from build123d import *

# Parameters (mm, degrees)
F1_DEPTH       = 20
F3_DEPTH       = 16
F5_DEPTH       = 16
F7_DEPTH       = 16
F9_DEPTH       = 18
F10_R          = 2.5
F11_DEPTH      = 17.4049884739
F11_DEPTH_BACK = 16
F13_DEPTH      = 16


with BuildPart() as f1:
    # F0 (on Top) → F1 (new body)
    with BuildSketch(Plane.XY):
        with BuildLine():
            ThreePointArc((23.6854385647, -8), (24.6691706804, -4.0536425523), (25, 0))
            ThreePointArc((25, 0), (24.6691706804, 4.0536425523), (23.6854385647, 8))
            ThreePointArc((23.6854385647, 8), (17.6776695297, 17.6776695297), (8, 23.6854385647))
            ThreePointArc((8, 23.6854385647), (0, 25), (-8, 23.6854385647))
            ThreePointArc((-8, 23.6854385647), (-17.6776695297, 17.6776695297), (-23.6854385647, 8))
            ThreePointArc((-23.6854385647, 8), (-25, 0), (-23.6854385647, -8))
            ThreePointArc((-23.6854385647, -8), (-17.6776695297, -17.6776695297), (-8, -23.6854385647))
            ThreePointArc((-8, -23.6854385647), (0, -25), (8, -23.6854385647))
            ThreePointArc((8, -23.6854385647), (17.6776695297, -17.6776695297), (23.6854385647, -8))
        make_face()
        with BuildLine():
            ThreePointArc((23.6854385647, 8), (24.6691706804, 4.0536425523), (25, 0))
            ThreePointArc((25, 0), (24.6691706804, -4.0536425523), (23.6854385647, -8))
            Line((23.6854385647, -8), (96.1854385647, -8))
            ThreePointArc((96.1854385647, -8), (104.1854385647, 0), (96.1854385647, 8))
            Line((96.1854385647, 8), (23.6854385647, 8))
        make_face()
        with BuildLine():
            ThreePointArc((-8, 23.6854385647), (0, 25), (8, 23.6854385647))
            Line((8, 23.6854385647), (8, 96.1854385647))
            ThreePointArc((8, 96.1854385647), (0, 104.1854385647), (-8, 96.1854385647))
            Line((-8, 96.1854385647), (-8, 23.6854385647))
        make_face()
        with BuildLine():
            Line((8, -96.1854385647), (8, -23.6854385647))
            ThreePointArc((8, -23.6854385647), (0, -25), (-8, -23.6854385647))
            Line((-8, -23.6854385647), (-8, -96.1854385647))
            ThreePointArc((-8, -96.1854385647), (0, -104.1854385647), (8, -96.1854385647))
        make_face()
        with BuildLine():
            ThreePointArc((-23.6854385647, -8), (-25, 0), (-23.6854385647, 8))
            Line((-23.6854385647, 8), (-96.1854385647, 8))
            ThreePointArc((-96.1854385647, 8), (-104.1854385647, 0), (-96.1854385647, -8))
            Line((-96.1854385647, -8), (-23.6854385647, -8))
        make_face()
    extrude(amount=F1_DEPTH)

    # F2 (on face) → F3 (cut, through all)
    with BuildSketch(Plane.YZ.offset(8)):
        Polygon((104.6854385647, 20), (23.6854385647, 20), (104.6854385647, 3), align=None)
    extrude(amount=-F3_DEPTH, mode=Mode.SUBTRACT)

    # F4 (on face) → F5 (cut, through all)
    with BuildSketch(Plane(origin=(0, 8, 0), x_dir=(-1, 0, 0), z_dir=(0, 1, 0))):
        Polygon((104.6854385647, 20), (23.6854385647, 20), (104.6854385647, 3), align=None)
    extrude(amount=-F5_DEPTH, mode=Mode.SUBTRACT)

    # F6 (on face) → F7 (cut, through all)
    with BuildSketch(Plane(origin=(-8, 0, 0), x_dir=(0, -1, 0), z_dir=(-1, 0, 0))):
        Polygon((104.6854385647, 20), (23.6854385647, 20), (104.6854385647, 3), align=None)
    extrude(amount=-F7_DEPTH, mode=Mode.SUBTRACT)

    # F8 (on face) → F9 (cut)
    with BuildSketch(Plane.XY.offset(20)):
        Polygon((10.7409683065, 0), (-0.5727401924, 11.313708499), (-11.8864486914, 0), (-0.5727401924, -11.313708499), align=None)
    extrude(amount=-F9_DEPTH, mode=Mode.SUBTRACT)

    # F10 (on face) → F11 (cut, two sides)
    with BuildSketch(Plane(origin=(5.3704841533, -5.3704841533, 0), x_dir=(-0.7071067812, -0.7071067812, 0), z_dir=(-0.7071067812, 0.7071067812, 0))) as f11_sk:
        with Locations((0, 3.5)):
            Circle(F10_R)
    extrude(amount=-F11_DEPTH, mode=Mode.SUBTRACT)
    extrude(f11_sk.sketch, amount=F11_DEPTH_BACK, mode=Mode.SUBTRACT)

    # F12 (on face) → F13 (cut, through all)
    with BuildSketch(Plane.XZ.offset(8)):
        Polygon((104.6854385647, 20), (23.6854385647, 20), (104.6854385647, 3), align=None)
    extrude(amount=-F13_DEPTH, mode=Mode.SUBTRACT)


solid = f1.part
CAD build for the part. Positions are in the model's coordinates, mm. A direction names the side the tool comes from. Give positions to 0.01 mm unless a question says otherwise; leave off trailing zeros. Loops run counter-clockwise (first coordinate to the right, second up) from the corner with the lowest first, then second, coordinate; pieces in that order, holes last. Notation, with made-up numbers: M 27.5,9.5 L 55.5,9.5 A14 cw 55.5,14.5 Z; hole C 51.5,-26.75 d5. An arc over 180 degrees is marked long. One line per question, with ' | ' between items. Start each with the question number.
1. 3-axis set-ups, long thin cutter, end or side, ignore diameter. For faces 1 (the face through (8, 51, 8)), 2 (the face through (51, -8, 8)), 3 (the face through (-51, 8, 8)), 4 (the face through (-6.15, 5.736, 10.633)): which of +Z, -Z, +X, -X, +Y, -Y reach the whole face in a straight line?
2. Flat gauge pins, fed straight in: pin 1 (6 mm diameter, centred on x = -50, z = 7, fed in from -Y); pin 2 (6 mm diameter, centred on x = -13, y = -52, fed in from +Z); pin 3 (3 mm diameter, centred on x = 78.5, z = 4, fed in from +Y); pin 4 (10 mm diameter, centred on y = 58.5, z = 6.5, fed in from +X). Where does each tip first touch, or does it go through?
3. Saw through at A-A on z = 17. Give the cut face in (x, y).
4. Saw through at C-C on x = 48. Give the cut face in (y, z).
5. Saw through at B-B on y = 89. Give the cut face in (x, z), plus the area to 3 significant figures.
6. Probe L1, parallel to X at y = -78, z = 8.25; L2, parallel to Y at x = -18, z = 2.5. List the from-to ranges inside material, lowest first. Write a range as from..to.
7. Two-plate mould, pull along Y, no slides. Class faces 5 (the face through (-17.564, 17.791, 9.86)), 6 (the face through (-52, -8, 8)), 7 (the face through (-8, -51, 8)), 8 (the face through (5, -5.74, 11.13)): pulls with the +Y half, pulls with the -Y half, needs draft (parallel to the pull), parting line crosses it, or undercut.
Result sheet:
1) face 1: +Z, -Z, +X, +Y | face 2: +Z, -Z, +X, -Y | face 3: +Z, -Z, -X, +Y | face 4: +Z
2) pin 1: stops at y = -8 | pin 2: passes through | pin 3: stops at y = 8 | pin 4: stops at x = 8
3) outline: M -37.98,-8 L -23.69,-8 A25 ccw -8,-23.69 L -8,-37.98 L 8,-37.98 L 8,-23.69 A25 ccw 23.69,-8 L 37.98,-8 L 37.98,8 L 23.69,8 A25 ccw 8,23.69 L 8,37.98 L -8,37.98 L -8,23.69 A25 ccw -23.69,8 L -37.98,8 Z; hole M -11.89,0 L -0.57,-11.31 L 10.74,0 L -0.57,11.31 Z
4) outline: M -8,0 L 8,0 L 8,14.9 L -8,14.9 Z
5) outline: M -8,0 L 8,0 L 8,6.29 L -8,6.29 Z | area: 101 mm^2
6) L1: x = -8..8 | L2: y = -17.35..17.35
7) face 5: pulls with the +Y half | face 6: pulls with the -Y half | face 7: needs draft | face 8: undercut
